CAD build for the part. Positions are in the model's coordinates, mm. A direction names the side the tool comes from. Coordinates: 2 decimals unless noted, no trailing zeros. Loops run counter-clockwise (first coordinate to the right, second up) from the corner with the lowest first, then second, coordinate; pieces in that order, holes last. Notation, with made-up numbers: (-10.5, 72) -> (30.5, 72) arc R27 ccw to (30.5, 95) -> close; hole circle Ø7 at (79.5, 29.25). An arc over 180 degrees is marked (long way). Answer as a JSON object with one key per item and string values. Group by question number.
from build123d import *

# Parameters (mm, degrees)
SKETCH1_R           = 7.1
BOSS_EXTRUDE1_DEPTH = 10.5
SKETCH2_R           = 11.5
BOSS_EXTRUDE2_DEPTH = 1
SKETCH3_R           = 3.175
CUT_EXTRUDE1_DEPTH  = 12.5


with BuildPart() as part:
    # Sketch1 → Boss-Extrude1 (new body)
    with BuildSketch(Plane(origin=(0, 0, 0), x_dir=(1, 0, 0), z_dir=(0, 1, 0))):
        Circle(SKETCH1_R)
    extrude(amount=BOSS_EXTRUDE1_DEPTH)

    # Sketch2 → Boss-Extrude2 (add)
    with BuildSketch(Plane(origin=(0, 10.5, 0), x_dir=(1, 0, 0), z_dir=(0, 1, 0))):
        Circle(SKETCH2_R)
    extrude(amount=BOSS_EXTRUDE2_DEPTH)

    # Sketch3 → Cut-Extrude1 (cut, through all)
    with BuildSketch(Plane.XZ):
        Circle(SKETCH3_R)
    extrude(amount=-CUT_EXTRUDE1_DEPTH, mode=Mode.SUBTRACT)


solid = part.part
Item 1: Pull direction X, two halves, no side cores. Call faces 1 (the flat face through (2.4, 11.5, 2.4)), 2 (the cylindrical face through (-0.69, 5.67, -3.1)), 3 (the cylindrical face through (-1.5, 11, -11.4)): +X half, -X half, draft (parallel to the pull), parting line (faces both ways), or undercut.
Item 2: Band-saw the part on D-D, the plane x = 4. List the corners of the cut face in (y, z).
Item 3: Band-saw the part on B-B, the plane x = 0. List the corners of the cut face in (y, z) (3 decimals).
Item 4: Drill centre lines: L1, parallel to Z at x = 0, y = 6 (3 decimals); L2, parallel to Z at x = -1.25, y = 0.5; L3, parallel to Y at x = -9, z = 1.5. Where is each one in solid material? Low to high.
Item 5: Band-saw the part on C-C, the plane y = 6.75. List the corners of the cut face in (x, z) (3 decimals), and give its area (3 significant figures).
Item 6: Band-saw the part on A-A, the plane z = 0. List the corners of the cut face in (x, y) (3 decimals).
Item 7: Flat gauge pins, fed straight in: P1, Ø5, axis at x = -2, y = 3, coming from the -Z side; P2, Ø3, axis at y = 3.5, z = -3, coming from the -X side; P3, Ø4, axis at y = 9, z = -2, coming from the +X side. Where does each tip first touch, or does it go through?
Item 8: 3-axis set-ups, long thin cutter, end or side, ignore diameter. For faces 4 (the flat face through (3.1, 0, 1.5)), 5 (the flat face through (5, 10.5, -5.3)): which of +Z, -Z, +X, -X, +Y, -Y reach the whole face in a straight line?
Reply:
{
 "1": {"face 1": "draft", "face 2": "undercut", "face 3": "parting line"},
 "2": {"outline": "(0, -5.87) -> (10.5, -5.87) -> (10.5, -10.78) -> (11.5, -10.78) -> (11.5, 10.78) -> (10.5, 10.78) -> (10.5, 5.87) -> (0, 5.87) -> close"},
 "3": {"outline": "(0, -7.1) -> (10.5, -7.1) -> (10.5, -11.5) -> (11.5, -11.5) -> (11.5, -3.175) -> (0, -3.175) -> close; (0, 3.175) -> (11.5, 3.175) -> (11.5, 11.5) -> (10.5, 11.5) -> (10.5, 7.1) -> (0, 7.1) -> close"},
 "4": {"L1": "-7.1 to -3.175, 3.175 to 7.1", "L2": "-6.99 to -2.92, 2.92 to 6.99", "L3": "10.5 to 11.5"},
 "5": {"outline": "circle Ø14.2 at (0, 0); hole circle Ø6.35 at (0, 0)", "area": "127 mm²"},
 "6": {"outline": "(-11.5, 10.5) -> (-7.1, 10.5) -> (-7.1, 0) -> (-3.175, 0) -> (-3.175, 11.5) -> (-11.5, 11.5) -> close; (3.175, 0) -> (7.1, 0) -> (7.1, 10.5) -> (11.5, 10.5) -> (11.5, 11.5) -> (3.175, 11.5) -> close"},
 "7": {"P1": "z = -7.1", "P2": "x = -6.94", "P3": "x = 11.48"},
 "8": {"face 4": "+Z, -Z, +X, -X, -Y", "face 5": "-Y"}
}
